Design review of the part built by this model. Coordinates are the model's own, in mm. Face numbers are marked on the shaded views. Give positions to 0.01 mm unless a question says otherwise; leave off trailing zeros. Write each loop counter-clockwise with the first axis right and the second up, starting at its lowest first coordinate (ties: lowest second). Pieces come first, ordered by that corner, then holes. Notation, with made-up numbers: (-31.5, 3.25) -> (2.5, 3.25) arc R19 ccw to (2.5, 16.25) -> close; hole circle Ø2 at (52, 32.25). An arc over 180 degrees is marked (long way). Put each result on its own line as item: value. Start each with the question number.
from build123d import *

# Parameters (mm, degrees)
CYLINDER003_R     = 3
CYLINDER003_DEPTH = 3
CYLINDER001_R     = 9.5
CYLINDER001_DEPTH = 10
CYLINDER_R        = 11.5
CYLINDER_DEPTH    = 3
CYLINDER002_R     = 3
CYLINDER002_DEPTH = 3


with BuildPart() as obj1:
    # Cylinder003 → Cylinder003 (new body)
    with BuildSketch(Plane(origin=(9, 9, 0), x_dir=(1, 0, 0), z_dir=(0, 0, 1))):
        Circle(CYLINDER003_R)
    extrude(amount=CYLINDER003_DEPTH)


with BuildPart() as cilindro_interior:
    # Cylinder001 → Cylinder001 (new body)
    with BuildSketch(Plane.XY.offset(-4)):
        Circle(CYLINDER001_R)
    extrude(amount=CYLINDER001_DEPTH)


with BuildPart() as obj2:
    # Cylinder → Cylinder (new body)
    with BuildSketch(Plane.XY):
        Circle(CYLINDER_R)
    extrude(amount=CYLINDER_DEPTH)

    # Cut: cut Cilindro-interior
    add(cilindro_interior.part, mode=Mode.SUBTRACT)


with BuildPart() as obj3:
    # Cylinder002 → Cylinder002 (new body)
    with BuildSketch(Plane(origin=(-9, 9, 0), x_dir=(1, 0, 0), z_dir=(0, 0, 1))):
        Circle(CYLINDER002_R)
    extrude(amount=CYLINDER002_DEPTH)

    # Fusion: union obj1, obj2
    add(obj1.part)
    add(obj2.part)


solid = obj3.part
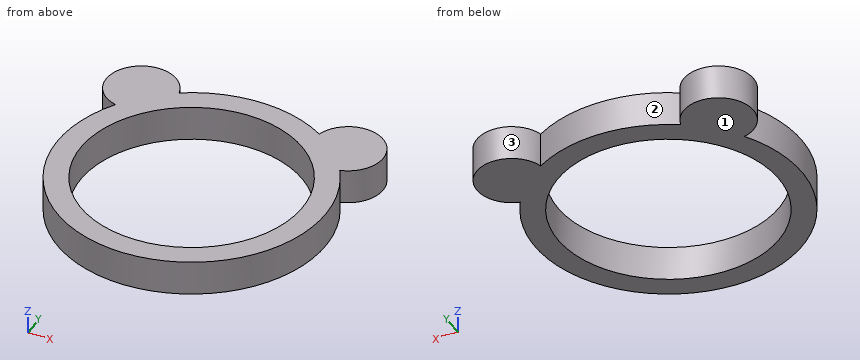
Q1. Mouldability with a two-part tool opening along X and no side actions: class the marked faces 1, 2 and 3 as +X half, -X half, draft (parallel to the pull), parting line (faces both ways), or undercut.
Q2. Take a section at C-C on z = 1.6. Give the boundary of the cut face in (x, y).
Q3. To check wall thickness, follow probe 1 along X at (y, z) = (0, 2); probe 2 along Y at (x, z) = (6.75, 2.35); probe 3 along X at (y, z) = (-7.75, 2.4). State the ranges of each line that lie inside material, in increasing order. Write a range as from..to.
Q4. For pin 1 (1.5 mm diameter, centred on x = -8.5, y = 0, fed in from -Z); pin 2 (1 mm diameter, centred on x = 5.5, z = 1, fed in from +Y), all flat-tipped, find the tip position at first contact; note any pin that passes through.
Q5. Take a section at A-A on y = 0. Give the boundary of the cut face in (x, z), then the cut area to 3 significant figures.
Result:
1. face 1: draft
1. face 2: undercut
1. face 3: undercut
2. outline: (-9.75, 6.1) arc R11.5 ccw (long way) to (9.75, 6.1) arc R3 ccw (long way) to (6.1, 9.75) arc R11.5 ccw to (-6.1, 9.75) arc R3 ccw (long way) to start; hole circle Ø19 at (0, 0)
3. probe 1: x = -11.5..-9.5, 9.5..11.5
3. probe 2: y = -9.31..-6.68, 6.68..10.98
3. probe 3: x = -8.5..-5.49, 5.49..8.5
4. pin 1: passes through
4. pin 2: stops at y = 10.36
5. outline: (-11.5, 0) -> (-9.5, 0) -> (-9.5, 3) -> (-11.5, 3) -> close; (9.5, 0) -> (11.5, 0) -> (11.5, 3) -> (9.5, 3) -> close
5. area: 12.0 mm^2
